Autodesk Inventor part; units mm, degrees
ref_plane "Work Plane1" through (23, -107, 0) normal (1, 0, 0) x (0, 0, 1)
ref_plane "YZ Plane" through (0, 0, 0) normal (1, 0, 0) x (0, 1, 0)
ref_plane "XZ Plane" through (0, 0, 0) normal (0, 1, 0) x (-1, 0, 0)
sketch "Sketch3" plane through (0, 0, 0) normal (0, 0, 1) x (1, 0, 0)
  line L0 (41.55, 0) -> (41.55, -24)
  line L1 (41.55, -24) -> (33, -107)
  line L2 (33, -107) -> (23, -107)
  line L3 (23, -107) -> (31.55, -24)
  line L4 (31.55, -24) -> (31.55, 0)
  line L5 (31.55, 0) -> (41.55, 0)
  line L6 (-8.31, 0) -> (49.86, 0)
  point P0 (0, 0)
  dimension "barWidth" = 10
  dimension "d33" = 24
  dimension "d37" = 23
  dimension "d38" = 41.55
  dimension "d39" = 107
extrude "Extrusion2" add sketch "Sketch3" along normal blind 20
ref_plane "Work Plane1" through (23, -107, 0) normal (1, 0, 0) x (0, 0, 1)
sketch "Sketch4" plane through (23, -107, 0) normal (1, 0, 0) x (0, 0, 1)
  arc A0 (-18.4663, 28.3548) -> (-25.5337, 9.6452) centre (-22, 19) ccw
  line L0 (-25.5337, 9.6452) -> (0, 0)
  line L1 (20, 0) -> (0, 0)
  line L2 (0, 0) -> (20, 0)
  line L3 (-22, 19) -> (-7.9678, 13.6994) construction
  line L4 (-23.4135, 15.2581) -> (-9.3812, 9.9575)
  line L5 (-6.5543, 17.4414) -> (-20.5865, 22.7419)
  arc A1 (-20.5865, 22.7419) -> (-23.4135, 15.2581) centre (-22, 19) ccw
  arc A2 (-9.3812, 9.9575) -> (-6.5543, 17.4414) centre (-7.9678, 13.6994) ccw
  line L6 (20, 0) -> (20, 13.8245)
  line L7 (20, 13.8245) -> (-18.4663, 28.3548)
  line L8 (20, 0) -> (20, -83)
  line L9 (0, -83) -> (0, 0)
  point P0 (0, -107)
  point P1 (-14.9839, 16.3497)
  dimension "d23" = 15
  dimension "d40" = 8
  dimension "d41" = 20
  dimension "d42" = 20
  dimension "d43" = 22
extrude "Extrusion4" add sketch "Sketch4" along normal blind 10
fillet "Fillet1" radius 2 2 edges at (36.55, 0, 20) (36.55, 0, 0)
sketch "Sketch5" plane through (41.55, -24, 20) normal (1, 0, 0) x (0, 0, -1)
  circle A0 centre (10, 14) radius 5.5
  line L0 (20, 22) -> (20, 0)
  line L1 (0, 0) -> (0, 22)
  line L2 (18, 24) -> (2, 24)
  point P0 (20, 24)
  dimension "d29" = 11
  dimension "d30" = 20
  dimension "d31" = 10
  dimension "d32" = 10
extrude "Extrusion5" cut sketch "Sketch5" against normal up to next
fillet "Fillet2" radius 8.25 1 edges at (28, -120.8245, 20)
fillet "Fillet3" radius 32.5 2 edges at (41.55, -24, 10) (31.55, -24, 10)
mirror "Mirror1" about plane through (0, 0, 0) normal (1, 0, 0)
sketch "Sketch6" plane through (0, 0, 20) normal (0, 0, 1) x (1, 0, 0)
  line L0 (70, -82.2581) -> (-70, -82.2581)
  line L1 (-70, -82.2581) -> (-70, -77.2581)
  line L2 (-70, -77.2581) -> (70, -77.2581)
  line L3 (70, -77.2581) -> (70, -82.2581)
  line L4 (33, -122.2581) -> (33, -130)
  point P0 (0, 0)
  point P1 (33, -129.7419)
  dimension "d46" = 140
  dimension "d47" = 5
  dimension "d48" = 70
  dimension "d57" = 40
extrude "Extrusion6" add sketch "Sketch6" along normal blind 60
fillet "Fillet4" radius 45.5 2 edges at (31.0638, -77.2581, 20) (-31.0638, -77.2581, 20)
fillet "Fillet5" radius 6 4 edges at (70, -79.7581, 20) (70, -79.7581, 80) (-70, -79.7581, 80) (-70, -79.7581, 20)
equation "\"d41\" = d42"
equation "\"d24\" = barWidth"
equation "\"d31\" = 0.5 * d30"
equation "\"d27\" = barWidth"
properties part number "AUX_batterry_mount"
Part model, mm, in its own coordinate system. A direction names the side the tool comes from. Round coordinates to 2 decimals unless told otherwise and drop trailing zeros. Write each loop counter-clockwise with the first axis right and the second up, starting at its lowest first coordinate (ties: lowest second). Pieces come first, ordered by that corner, then holes. Notation, with made-up numbers: (65.25, 89.5) -> (106.25, 89.5) arc R15 ccw to (106.25, 111.5) -> close; hole circle Ø1 at (1.5, 34). An arc over 180 degrees is marked (long way). Return JSON: item names as keys, results as strings. Group by question number.
Q1. Which spindle directions (+Z, -Z, +X, -X, +Y, -Y) get a long thin tool onto all of the face, cutting with end or side? Do faces 1 (the flat face through (-31.55, -16, 10)), 2 (the flat face through (27.93, -119.645, -16.496)), 3 (the flat face through (-32, -54, 0)), 4 (the cylindrical face through (33.5, -64.3, 33.7)), 5 (the flat face through (50, -80, 20)). Say none if no direction does.
Q2. Probe L1, parallel to X at y = -104, z = 19; L2, parallel to Y at x = 56, z = 64.5; L3, parallel to X at y = -77.5, z = 19. List the from-to ranges inside material, lowest first. Write a range as [from, to].
Q3. Saw through at B-B on y = -10. Write the cut outline in (x, z).
Q4. Pin check, flat tips, straight feed: pin 1 (15 mm diameter, centred on x = 28, y = -56, fed in from -Z); pin 2 (6.5 mm diameter, centred on x = -31, y = -98, fed in from +Z); pin 3 (4 mm diameter, centred on y = -17, z = 21, fed in from +X). Stop position of each tip, or through.
Q5. Mould opens along Y. For faces 6 (the flat face through (-70, -80, 50)), 7 (the cylindrical face through (36.6, -14.9, 7.5)), 8 (the flat face through (-37.13, -66.9, 17.74)), 9 (the flat face through (36, 0, 10)) say: pulls with the +Y half, pulls with the -Y half, needs draft (parallel to the pull), parting line crosses it, or undercut.
Q6. Saw through at C-C on y = -36.5. Write the cut outline in (x, z), plus the area to 3 significant figures.
Q7. Saw through at D-D on x = 1. Write the cut outline in (y, z).
Q8. Saw through at A-A on z = 10. Write the cut outline in (x, y), plus the area to 3 significant figures.
Answer:
{
 "1": {"face 1": "+Z, -Z, +Y", "face 2": "+X, -X", "face 3": "-Z, +X, -X, +Y", "face 4": "+Z, +X, -X, +Y", "face 5": "-Z, +X, -Y"},
 "2": {"L1": "[-33.31, -23.31], [23.31, 33.31]", "L2": "[-82.26, -77.26]", "L3": "[-36.04, -26.04], [26.04, 36.04]"},
 "3": {"outline": "(-41.55, 0) -> (-31.55, 0) -> (-31.55, 4.5) -> (-41.55, 4.5) -> close; (-41.55, 15.5) -> (-31.55, 15.5) -> (-31.55, 20) -> (-41.55, 20) -> close; (31.55, 0) -> (41.55, 0) -> (41.55, 4.5) -> (31.55, 4.5) -> close; (31.55, 15.5) -> (41.55, 15.5) -> (41.55, 20) -> (31.55, 20) -> close"},
 "4": {"pin 1": "z = 0", "pin 2": "z = 20", "pin 3": "x = 41.55"},
 "5": {"face 6": "needs draft", "face 7": "undercut", "face 8": "undercut", "face 9": "pulls with the +Y half"},
 "6": {"outline": "(-40.26, 0) -> (-30.26, 0) -> (-30.26, 20.25) -> (-40.26, 20.25) -> close; (30.26, 0) -> (40.26, 0) -> (40.26, 20.25) -> (30.26, 20.25) -> close", "area": "405 mm2"},
 "7": {"outline": "(-82.26, 20) -> (-77.26, 20) -> (-77.26, 80) -> (-82.26, 80) -> close"},
 "8": {"outline": "(-41.55, -22.33) arc R32.5 ccw to (-41.38, -25.66) -> (-33, -107) -> (-33, -124.6) -> (-23, -124.6) -> (-23, -107) -> (-31.38, -25.66) arc R32.5 cw to (-31.55, -22.33) -> (-31.55, -15.5) -> (-41.55, -15.5) -> close; (-41.55, -4.5) -> (-31.55, -4.5) -> (-31.55, 0) -> (-41.55, 0) -> close; (23, -124.6) -> (33, -124.6) -> (33, -107) -> (41.38, -25.66) arc R32.5 ccw to (41.55, -22.33) -> (41.55, -15.5) -> (31.55, -15.5) -> (31.55, -22.33) arc R32.5 cw to (31.38, -25.66) -> (23, -107) -> close; (31.55, -4.5) -> (41.55, -4.5) -> (41.55, 0) -> (31.55, 0) -> close", "area": "2,270 mm2"}
}
